Check sheet for the modelled part. Datum: model origin and axes. Units: mm. Round coordinates to 2 decimals unless told otherwise and drop trailing zeros. Loops run counter-clockwise (first coordinate to the right, second up) from the corner with the lowest first, then second, coordinate; pieces in that order, holes last. Notation, with made-up numbers: (84, 67) -> (99, 67) arc R24 cw to (99, 84) -> close; hole circle Ø4 at (-29.5, 11). An arc over 180 degrees is marked (long way). Return JSON: item names as keys, results as strings.
from build123d import *

# Parameters (mm, degrees)
SKETCH_1_W          = 5
SKETCH_1_H          = 15
EXTRUDE_1_DEPTH     = 5
SKETCH_2_R          = 1.3
SKETCH_2_R_2        = 1.2
SKETCH_2_R_3        = 1.1
CUT_EXTRUDE_1_DEPTH = 5


with BuildPart() as part:
    # 草图1 → 凸台-拉伸1 (new body)
    with BuildSketch(Plane(origin=(0, 0, 0), x_dir=(1, 0, 0), z_dir=(0, 1, 0))):
        with Locations((-10.380434783, -6.711956522)):
            Rectangle(SKETCH_1_W, SKETCH_1_H)
    extrude(amount=EXTRUDE_1_DEPTH)

    # 草图2 → 切除-拉伸1 (cut)
    with BuildSketch(Plane(origin=(0, 5, 0), x_dir=(1, 0, 0), z_dir=(0, 1, 0))):
        with Locations(Location((-10.380434783, -11.711956522, 0), (0, 0, 270))):
            Circle(SKETCH_2_R)
        with Locations(Location((-10.380434783, -7.02762262, 0), (0, 0, 270))):
            Circle(SKETCH_2_R_2)
        with Locations(Location((-10.380434783, -2.552955038, 0), (0, 0, 270))):
            Circle(SKETCH_2_R_3)
    extrude(amount=-CUT_EXTRUDE_1_DEPTH, mode=Mode.SUBTRACT)


solid = part.part
Q1. Section check C-C (x = -11.15). Record the boundary of the cut face in (y, z).
Results list:
{"outline": "(0, -0.79) -> (5, -0.79) -> (5, 1.77) -> (0, 1.77) -> close; (0, 3.34) -> (5, 3.34) -> (5, 6.11) -> (0, 6.11) -> close; (0, 7.95) -> (5, 7.95) -> (5, 10.66) -> (0, 10.66) -> close; (0, 12.76) -> (5, 12.76) -> (5, 14.21) -> (0, 14.21) -> close"}
Q2. Material ranges on line 1 (Z direction, x = -10.4, y = 4.5); line 2 (Z direction, x = -9.8, y = 4.3); line 3 (X direction, y = 3.05, z = 11), recorded low to high.
Results list:
{"line 1": "-0.79 to 1.45, 3.65 to 5.83, 8.23 to 10.41, 13.01 to 14.21", "line 2": "-0.79 to 1.62, 3.49 to 5.98, 8.08 to 10.55, 12.88 to 14.21", "line 3": "-12.88 to -11.47, -9.29 to -7.88"}
Q3. Section check A-A (z = 6.5). Record the boundary of the cut face in (x, y).
Results list:
{"outline": "(-12.88, 0) -> (-11.46, 0) -> (-11.46, 5) -> (-12.88, 5) -> close; (-9.3, 0) -> (-7.88, 0) -> (-7.88, 5) -> (-9.3, 5) -> close"}
Q4. Draft check along X on faces 1 (the cylindrical face through (-9.29, 2.54, 2.41)), 2 (the flat face through (-12.88, 2, 7)), 3 (the cylindrical face through (-10.323, 2.535, 10.413)), 4 (the flat face through (-7.88, 2, 7)). Enter one of: released by +X, released by -X, zero draft, split by the parting line, or undercut.
Results list:
{"face 1": "undercut", "face 2": "released by -X", "face 3": "undercut", "face 4": "released by +X"}
Q5. Section check B-B (y = 1.5). Record the boundary of the cut face in (x, z), then the cut area to 3 significant figures.
Results list:
{"outline": "(-12.88, -0.79) -> (-7.88, -0.79) -> (-7.88, 14.21) -> (-12.88, 14.21) -> close; hole circle Ø2.6 at (-10.38, 11.71); hole circle Ø2.4 at (-10.38, 7.03); hole circle Ø2.2 at (-10.38, 2.55)", "area": "61.4 mm^2"}
Q6. Section check D-D (z = 2). Record the boundary of the cut face in (x, y).
Results list:
{"outline": "(-12.88, 0) -> (-11.33, 0) -> (-11.33, 5) -> (-12.88, 5) -> close; (-9.43, 0) -> (-7.88, 0) -> (-7.88, 5) -> (-9.43, 5) -> close"}
